```python
from build123d import *


with BuildPart() as f1:
    # F0 (on Front) → F1 (revolve)
    with BuildSketch(Plane.XZ):
        with BuildLine():
            Line((-5, 0), (-2, 0))
            Line((-2, 0), (-2, 7))
            Line((-2, 7), (-4, 9))
            Line((-4, 9), (-4, 10))
            Line((-4, 10), (-6, 10))
            ThreePointArc((-6, 10), (-6.707107, 9.707107), (-7, 9))
            Line((-7, 9), (-7, 8))
            ThreePointArc((-7, 8), (-6.707107, 7.292893), (-6, 7))
            Line((-6, 7), (-4, 7))
            ThreePointArc((-4, 7), (-3.646447, 6.853553), (-3.5, 6.5))
            Line((-3.5, 6.5), (-3.5, 2.5))
            ThreePointArc((-3.5, 2.5), (-3.93934, 1.43934), (-5, 1))
            Line((-5, 1), (-5, 0))
        make_face()
    revolve(axis=Axis((0, 0, -0.231959), (0, 0, -1)))


solid = f1.part
```
Geometry: final body of the model. Coordinates: model frame, mm. A direction names the side the tool comes from. Coordinates: 2 decimals unless noted, no trailing zeros. Loops run counter-clockwise (first coordinate to the right, second up) from the corner with the lowest first, then second, coordinate; pieces in that order, holes last. Notation, with made-up numbers: M 65,-27.5 L 94,-27.5 A19 ccw 94,-17.5 Z; hole C -5,20.25 d4. An arc over 180 degrees is marked long. Put each result on its own line as item: value.
(1) Material intervals for probe 1 along Y at (x, z) = (0, 3.5); probe 2 along Z at (x, y) = (2.5, 4.5); probe 3 along Y at (x, z) = (-1, 8.75), sorted ascending.
Answer sheet:
probe 1: y = -3.5 to -2, 2 to 3.5
probe 2: z = 7 to 10
probe 3: y = -6.93 to -3.61, 3.61 to 6.93
(2) Cut plane D-D on z = 8.25. Return the cut outline in (x, y), then the cut area to 3 significant figures.
Answer sheet:
outline: C 0,0 d14; hole C 0,0 d6.5
area: 121 mm^2
(3) First-contact query: pin 1 (5 mm diameter, centred on y = -4.5, z = 4, fed in from +X). Flat tip, straight axial feed; report the tip coordinate or a pass-through.
Answer sheet:
pin 1: stops at x = 2.87
(4) Cut plane C-C on z = 3.75. Return the cut outline in (x, y), then the cut area to 3 significant figures.
Answer sheet:
outline: C 0,0 d7; hole C 0,0 d4
area: 25.9 mm^2
(5) Access query for faces 5 (the face through (2.123, 0.093, 7.125)), 6 (the face through (1.08, -4.88, 0.49)), 7 (the face through (1.42, -3.92, 7)). Directions: +Z, -Z, +X, -X, +Y, -Y. A direction counts if a zero-diameter tool reaches every point of the face in a straight line with its end or side. Return the directions, or none.
Answer sheet:
face 5: +Z
face 6: -Z
face 7: none
(6) Cut plane A-A on y = 0. Return the cut outline in (x, z), then the cut area to 3 significant figures.
Answer sheet:
outline: M -7,8 A1 ccw -6,7 L -4,7 A0.5 cw -3.5,6.5 L -3.5,2.5 A1.5 cw -5,1 L -5,0 L -2,0 L -2,7 L -4,9 L -4,10 L -6,10 A1 ccw -7,9 Z; M 2,0 L 5,0 L 5,1 A1.5 cw 3.5,2.5 L 3.5,6.5 A0.5 cw 4,7 L 6,7 A1 ccw 7,8 L 7,9 A1 ccw 6,10 L 4,10 L 4,9 L 2,7 Z
area: 46.2 mm^2
(7) Draft query along Z for faces 1 (the face through (0.867, -3.905, 9.507)), 2 (the face through (-1.42, -3.92, 10)), 3 (the face through (-2.2, 0.1, 0)), 4 (the face through (-3.233, -1.341, 4.472)). Return one class per face: pulls with the +Z half, pulls with the -Z half, needs draft (parallel to the pull), parting line crosses it, or undercut.
Answer sheet:
face 1: needs draft
face 2: pulls with the +Z half
face 3: pulls with the -Z half
face 4: undercut
